Model file for the job. Use its own axes, mm. A direction names the side the tool comes from. Give positions to 0.01 mm unless a question says otherwise; leave off trailing zeros. Loops run counter-clockwise (first coordinate to the right, second up) from the corner with the lowest first, then second, coordinate; pieces in that order, holes last. Notation, with made-up numbers: (68, 9.25) - (118, 9.25) arc R22 ccw to (118, 18.25) - close; hole circle Ø9 at (53, 12.5). An arc over 180 degrees is marked (long way). Use a Markdown table: item, result.
from build123d import *

# Parameters (mm, degrees)
SKETCH_1_R               = 11.5
SKETCH_1_R_2             = 1.75
SKETCH_1_R_3             = 2.5
SKETCH_1_R_4             = 3.6
SM_BASE_FLANGE_1_DEPTH   = 2
SKETCH_4_R               = 3.25
EXTRUDE_1_DEPTH          = 2
HOLE_WIZARD_M3_2_D       = 2.5
CUT_EXTRUDE_1_REACH      = 86.132
SKETCH_8_R               = 2.1
EXTRUDE_2_DEPTH          = 12
HOLE_WIZARD_M2_5_1_D     = 2.05
HOLE_WIZARD_M2_5_1_DEPTH = 10
CUT_EXTRUDE_2_REACH      = 86.89
SKETCH_11_R              = 1.6
SKETCH_12_R              = 3.25
EXTRUDE_3_DEPTH          = 2
HOLE_WIZARD_M3_3_D       = 2.5
CUT_EXTRUDE_3_REACH      = 87.195
SKETCH_15_R              = 1.5


# Sheet-metal steps are written as plain solids
with BuildPart() as part:
    # Sketch 1 → 基体-法兰1 (new body)
    with BuildSketch(Plane.XY):
        with BuildLine():
            Line((-1.743446796, -45.5), (31.707432394, -45.5))
            ThreePointArc((31.707432394, -45.5), (32.958860234, -45.340860292), (34.130627329, -44.873571345))
            Line((34.130627329, -44.873571345), (62.269584803, -29.283067879))
            ThreePointArc((62.269584803, -29.283067879), (67.923694751, -23.776689927), (70, -16.162353844))
            Line((70, -16.162353844), (70, -5))
            ThreePointArc((70, -5), (65.606601718, 5.606601718), (55, 10))
            Line((55, 10), (31, 10))
            ThreePointArc((31, 10), (16.857864376, 15.857864376), (11, 30))
            Line((11, 30), (11, 35.5))
            ThreePointArc((11, 35.5), (5.079234746, 45.257119165), (-6.3093408, 44.510672487))
            Line((-6.3093408, 44.510672487), (-20.879582297, 34.308479557))
            ThreePointArc((-20.879582297, 34.308479557), (-23.608288666, 32.962830493), (-26.615346661, 32.5))
            Line((-26.615346661, 32.5), (-57, 32.5))
            ThreePointArc((-57, 32.5), (-59.121320344, 31.621320344), (-60, 29.5))
            Line((-60, 29.5), (-60, -29.5))
            ThreePointArc((-60, -29.5), (-59.121320344, -31.621320344), (-57, -32.5))
            Line((-57, -32.5), (-26.615346661, -32.5))
            ThreePointArc((-26.615346661, -32.5), (-23.608288666, -32.962830493), (-20.879582297, -34.308479557))
            Line((-20.879582297, -34.308479557), (-7.479211159, -43.691520443))
            ThreePointArc((-7.479211159, -43.691520443), (-4.750504791, -45.037169507), (-1.743446796, -45.5))
        make_face()
        with Locations((-38, 0)):
            Circle(SKETCH_1_R, mode=Mode.SUBTRACT)
        with Locations((-22.5, 15.5)):
            Circle(SKETCH_1_R_2, mode=Mode.SUBTRACT)
        with Locations(Location((-22.5, -15.5, 0), (0, 0, 180))):
            Circle(SKETCH_1_R_2, mode=Mode.SUBTRACT)
        with Locations((0, 35.5)):
            Circle(SKETCH_1_R_3, mode=Mode.SUBTRACT)
        with Locations(Location((0, -35.5, 0), (0, 0, 180))):
            Circle(SKETCH_1_R_3, mode=Mode.SUBTRACT)
        with Locations((-53.5, -15.5)):
            Circle(SKETCH_1_R_2, mode=Mode.SUBTRACT)
        with Locations(Location((-53.5, 15.5, 0), (0, 0, 180))):
            Circle(SKETCH_1_R_2, mode=Mode.SUBTRACT)
        with Locations((60, -12)):
            Circle(SKETCH_1_R_4, mode=Mode.SUBTRACT)
    extrude(amount=-SM_BASE_FLANGE_1_DEPTH)

    # 草图4 → 凸台-拉伸1 (add)
    with BuildSketch(Plane(origin=(0, 0, -2), x_dir=(-1, 0, 0), z_dir=(0, 0, -1))):
        with Locations((-10, 0)):
            Circle(SKETCH_4_R)
        with Locations((-35, 0)):
            Circle(SKETCH_4_R)
    extrude(amount=EXTRUDE_1_DEPTH)

    # M3 螺纹孔2 (through all)
    with Locations(Plane(origin=(0, 0, 0), x_dir=(-1, 0, 0), z_dir=(0, 0, 1))):
        with Locations((-10, 0), (-35, 0)):
            Hole(HOLE_WIZARD_M3_2_D / 2)

    # 草图7 → 切除-拉伸1 (cut, up to next)
    with BuildSketch(Plane.XY, mode=Mode.PRIVATE) as cut_extrude_1_sk1:
        with BuildLine():
            Line((-38, 22.5), (-41, 22.5))
            ThreePointArc((-41, 22.5), (-42.5, 24), (-41, 25.5))
            Line((-41, 25.5), (-38, 25.5))
            ThreePointArc((-38, 25.5), (-36.5, 24), (-38, 22.5))
        make_face()
    cut_extrude_1_tool1 = extrude(cut_extrude_1_sk1.sketch, amount=-CUT_EXTRUDE_1_REACH, mode=Mode.PRIVATE) & part.part
    # 草图7 → 切除-拉伸1 (cut, up to next)
    with BuildSketch(Plane.XY, mode=Mode.PRIVATE) as cut_extrude_1_sk2:
        with BuildLine():
            Line((-38, -25.5), (-41, -25.5))
            ThreePointArc((-41, -25.5), (-42.5, -24), (-41, -22.5))
            Line((-41, -22.5), (-38, -22.5))
            ThreePointArc((-38, -22.5), (-36.5, -24), (-38, -25.5))
        make_face()
    cut_extrude_1_tool2 = extrude(cut_extrude_1_sk2.sketch, amount=-CUT_EXTRUDE_1_REACH, mode=Mode.PRIVATE) & part.part
    add(cut_extrude_1_tool1.solids().sort_by_distance((-39.5, 24, 0))[0], mode=Mode.SUBTRACT)
    add(cut_extrude_1_tool2.solids().sort_by_distance((-39.5, -24, 0))[0], mode=Mode.SUBTRACT)

    # 草图8 → 凸台-拉伸2 (add)
    with BuildSketch(Plane.XY):
        with Locations(Location((-23, 4.75, 0), (0, 0, 180))):
            Circle(SKETCH_8_R)
        with Locations(Location((-23, -4.75, 0), (0, 0, 180))):
            Circle(SKETCH_8_R)
    extrude(amount=EXTRUDE_2_DEPTH)

    # M2.5 螺纹孔1
    with Locations(Plane.XY.offset(12)):
        with Locations((-23, 4.75), (-23, -4.75)):
            Hole(HOLE_WIZARD_M2_5_1_D / 2, depth=HOLE_WIZARD_M2_5_1_DEPTH)

    # 草图11 → 切除-拉伸2 (cut, up to next)
    with BuildSketch(Plane.XY, mode=Mode.PRIVATE) as cut_extrude_2_sk1:
        with Locations((-51, 27.5)):
            Circle(SKETCH_11_R)
    cut_extrude_2_tool1 = extrude(cut_extrude_2_sk1.sketch, amount=-CUT_EXTRUDE_2_REACH, mode=Mode.PRIVATE) & part.part
    # 草图11 → 切除-拉伸2 (cut, up to next)
    with BuildSketch(Plane.XY, mode=Mode.PRIVATE) as cut_extrude_2_sk2:
        with Locations((-51, -27.5)):
            Circle(SKETCH_11_R)
    cut_extrude_2_tool2 = extrude(cut_extrude_2_sk2.sketch, amount=-CUT_EXTRUDE_2_REACH, mode=Mode.PRIVATE) & part.part
    add(cut_extrude_2_tool1.solids().sort_by_distance((-51, 27.5, 0))[0], mode=Mode.SUBTRACT)
    add(cut_extrude_2_tool2.solids().sort_by_distance((-51, -27.5, 0))[0], mode=Mode.SUBTRACT)

    # 草图12 → 凸台-拉伸3 (add)
    with BuildSketch(Plane.XY.offset(-2)):
        with Locations((26, -40.5)):
            Circle(SKETCH_12_R)
        with Locations((34, -40.5)):
            Circle(SKETCH_12_R)
    extrude(amount=-EXTRUDE_3_DEPTH)

    # M3 螺纹孔3 (through all)
    with Locations(Plane(origin=(0, 0, 0), x_dir=(-1, 0, 0), z_dir=(0, 0, 1))):
        with Locations((-34, 40.5), (-26, 40.5)):
            Hole(HOLE_WIZARD_M3_3_D / 2)

    # 草图15 → 切除-拉伸3 (cut, up to next)
    with BuildSketch(Plane(origin=(0, 0, -2), x_dir=(-1, 0, 0), z_dir=(0, 0, -1)), mode=Mode.PRIVATE) as cut_extrude_3_sk1:
        with Locations((15, -34.5)):
            Circle(SKETCH_15_R)
    cut_extrude_3_tool1 = extrude(cut_extrude_3_sk1.sketch, amount=-CUT_EXTRUDE_3_REACH, mode=Mode.PRIVATE) & part.part
    add(cut_extrude_3_tool1.solids().sort_by_distance((-15, -34.5, -2))[0], mode=Mode.SUBTRACT)


solid = part.part
(1) Slice it at A-A, the plane z = 7.75. Write the cut outline in (x, y) (3 decimals), plus the area to 3 significant figures.
Computed:
| item | result |
|---|---|
| outline | circle Ø4.2 at (-23, -4.75); circle Ø4.2 at (-23, 4.75); hole circle Ø2.05 at (-23, -4.75); hole circle Ø2.05 at (-23, 4.75) |
| area | 21.1 mm² |
(2) Slice it at C-C, the plane y = 27.5. Write the cut outline in (x, z).
Computed:
| item | result |
|---|---|
| outline | (-60, -2) - (-52.6, -2) - (-52.6, 0) - (-60, 0) - close; (-49.4, -2) - (11.16, -2) - (11.16, 0) - (-49.4, 0) - close |
(3) 3-axis set-ups, long thin cutter, end or side, ignore diameter. For faces 4 (the cylindrical face through (25.295, -43.673, -2.986)), 5 (the cylindrical face through (-23.969, 6.613, 5.916)), 6 (the cylindrical face through (-13.8, -35.4, -1)): which of +Z, -Z, +X, -X, +Y, -Y reach the whole face in a straight line?
Computed:
| item | result |
|---|---|
| face 4 | -Z |
| face 5 | +Z |
| face 6 | +Z, -Z |
(4) Drill centre lines: probe 1 along Y at (x, z) = (-51, -0.55); probe 2 along Y at (x, z) = (-53.5, -0.85); probe 3 along X at (y, z) = (-40.5, -1.2). Where is each one in solid material? Low to high. Write a range as [from, to].
Computed:
| item | result |
|---|---|
| probe 1 | [-32.5, -29.1], [-25.9, 25.9], [29.1, 32.5] |
| probe 2 | [-32.5, -17.25], [-13.75, 13.75], [17.25, 32.5] |
| probe 3 | [-12.04, 24.75], [27.25, 32.75], [35.25, 42.02] |
(5) Slice it at B-B, the plane x = 0. Write the cut outline in (y, z), plus the area to 3 significant figures.
Computed:
| item | result |
|---|---|
| outline | (-45.5, -2) - (-38, -2) - (-38, 0) - (-45.5, 0) - close; (-33, -2) - (33, -2) - (33, 0) - (-33, 0) - close; (38, -2) - (46.5, -2) - (46.5, 0) - (38, 0) - close |
| area | 164 mm² |
(6) Pin check, flat tips, straight feed: P1, Ø3.5, axis at x = -15, y = -34.5, coming from the -Z side; P2, Ø0.6, axis at x = -42.5, z = -1.5, coming from the +Y side; P3, Ø3, axis at x = -22.5, y = 15.5, coming from the +Z side; P4, Ø1, axis at x = -39, z = -1, coming from the -Y side. Stop position of each tip, or through.
Computed:
| item | result |
|---|---|
| P1 | z = -2 |
| P2 | y = 32.5 |
| P3 | through |
| P4 | y = -32.5 |
(7) Slice it at D-D, the plane x = -39.5. Write the cut outline in (y, z), plus the area to 3 significant figures.
Computed:
| item | result |
|---|---|
| outline | (-32.5, -2) - (-25.5, -2) - (-25.5, 0) - (-32.5, 0) - close; (-22.5, -2) - (-11.4, -2) - (-11.4, 0) - (-22.5, 0) - close; (11.4, -2) - (22.5, -2) - (22.5, 0) - (11.4, 0) - close; (25.5, -2) - (32.5, -2) - (32.5, 0) - (25.5, 0) - close |
| area | 72.4 mm² |
(8) Mould opens along Y. For faces 1 (the cylindrical face through (65.72, 5.49, -0.99)), 2 (the cylindrical face through (0.54, -33.06, -0.99)), 3 (the cylindrical face through (-59.14, -31.6, -0.99)) say: pulls with the +Y half, pulls with the -Y half, needs draft (parallel to the pull), parting line crosses it, or undercut.
Computed:
| item | result |
|---|---|
| face 1 | pulls with the +Y half |
| face 2 | undercut |
| face 3 | pulls with the -Y half |
